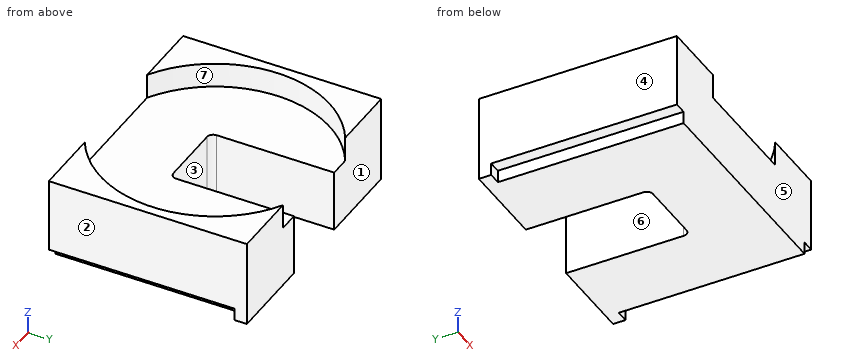
from build123d import *

# Parameters (mm, degrees)
F0_W          = 200
F0_H          = 160
F1_DEPTH      = 50
F3_DEPTH      = 20
F5_W          = 60
F5_H          = 120
F6_DEPTH      = 90
F6_DEPTH_BACK = 20
F9_W          = 10
F9_H          = 10
F10_DEPTH     = 150
F11_R         = 5


with BuildPart() as f1:
    # F0 (on Top) → F1 (new body)
    with BuildSketch(Plane.XY):
        Rectangle(F0_W, F0_H)
    extrude(amount=F1_DEPTH)

    # F2 (on face) → F3 (join)
    with BuildSketch(Plane.XY.offset(50)):
        with BuildLine():
            ThreePointArc((46.4354390525, 80), (80.1608636192, 46.1571873474), (92.5, 0))
            ThreePointArc((92.5, 0), (80.1608636192, -46.1571873474), (46.4354390525, -80))
            Line((46.4354390525, -80), (100, -80))
            Line((100, -80), (100, 80))
            Line((100, 80), (46.4354390525, 80))
        make_face()
        with BuildLine():
            ThreePointArc((-46.4354390525, -80), (-92.5, 0), (-46.4354390525, 80))
            Line((-46.4354390525, 80), (-100, 80))
            Line((-100, 80), (-100, -80))
            Line((-100, -80), (-46.4354390525, -80))
        make_face()
    extrude(amount=F3_DEPTH)

    # F5 (on Front) → F6 (cut, two sides)
    with BuildSketch(Plane.XZ) as f6_sk:
        Rectangle(F5_W, F5_H)
    extrude(amount=-F6_DEPTH, mode=Mode.SUBTRACT)
    extrude(f6_sk.sketch, amount=F6_DEPTH_BACK, mode=Mode.SUBTRACT)

    # F9 (on face) → F10 (cut)
    with BuildSketch(Plane.XZ.offset(80)):
        with Locations((95, 5)):
            Rectangle(F9_W, F9_H)
        with Locations((-95, 5)):
            Rectangle(F9_W, F9_H)
    extrude(amount=-F10_DEPTH, mode=Mode.SUBTRACT)

    # F11
    f11_edges = [f1.edges().sort_by_distance(p)[0] for p in [
        (-30, -20, 25),
        (30, -20, 25),
    ]]
    fillet(f11_edges, radius=F11_R)


solid = f1.part
Check sheet for the modelled part. Datum: model origin and axes. Units: mm. Face numbers are marked on the shaded views. A direction names the side the tool comes from. Round coordinates to 2 decimals unless told otherwise and drop trailing zeros. Loops run counter-clockwise (first coordinate to the right, second up) from the corner with the lowest first, then second, coordinate; pieces in that order, holes last.
1. Gauge pin test, flat ends, axial feed: pin 1 Ø11 at (y, z) = (8.5, 5.5) entering from -X; pin 2 Ø12 at (x, z) = (1, 12.5) entering from +Y; pin 3 Ø3 at (x, z) = (93.5, 3) entering from -Y; pin 4 Ø5 at (y, z) = (-31.5, 3.5) entering from +X. Record the tip position at first contact, or that the pin passes through.
2. Sectioned sample at B-B on y = 27. Record the boundary of the cut face in (x, z).
3. Sectioned sample at C-C on x = 85.5. Record the boundary of the cut face in (y, z).
4. Set-up check for the marked faces 5, 6 and 7: record each of +Z, -Z, +X, -X, +Y, -Y from which the full face is reachable in a straight line by a thin tool's end or side.
5. Scan lines: probe 1 along X at (y, z) = (-9.5, 12); probe 2 along Y at (x, z) = (68, 53); probe 3 along Z at (x, y) = (88.5, 10.5). Record each from-to range of solid material in increasing order.
6. Mould release check, pull along X, two halves, no side actions. Record for the marked faces 1, 2, 3 and 4: released by +X, released by -X, zero draft, split by the parting line, or undercut.
7. Sectioned sample at A-A on z = 54. Record the boundary of the cut face in (x, y).
8. Sectioned sample at D-D on y = -31. Record the boundary of the cut face in (x, z).
Recorded:
1. pin 1: stops at x = -100
1. pin 2: stops at y = -20
1. pin 3: stops at y = 70
1. pin 4: stops at x = 90
2. outline: (-100, 10) - (-90, 10) - (-90, 0) - (-30, 0) - (-30, 50) - (-88.47, 50) - (-88.47, 70) - (-100, 70) - close; (30, 0) - (90, 0) - (90, 10) - (100, 10) - (100, 70) - (88.47, 70) - (88.47, 50) - (30, 50) - close
3. outline: (-80, 0) - (80, 0) - (80, 70) - (35.3, 70) - (35.3, 50) - (-35.3, 50) - (-35.3, 70) - (-80, 70) - close
4. face 5: +Z, -Z, +X, -X, -Y
4. face 6: +Z, -Z, +Y
4. face 7: +Z
5. probe 1: x = -100 to -30, 30 to 100
5. probe 2: y = -80 to -62.71, 62.71 to 80
5. probe 3: z = 0 to 50
6. face 1: zero draft
6. face 2: released by +X
6. face 3: undercut
6. face 4: released by -X
7. outline: (-100, -80) - (-46.44, -80) arc R92.5 cw to (-46.44, 80) - (-100, 80) - close; (46.44, -80) - (100, -80) - (100, 80) - (46.44, 80) arc R92.5 cw to start
8. outline: (-100, 10) - (-90, 10) - (-90, 0) - (90, 0) - (90, 10) - (100, 10) - (100, 70) - (87.15, 70) - (87.15, 50) - (-87.15, 50) - (-87.15, 70) - (-100, 70) - close
